Work out the finished part from the listing and answer in its coordinate system (mm). A direction names the side the tool comes from. Round coordinates to 2 decimals unless told otherwise and drop trailing zeros. Loops run counter-clockwise (first coordinate to the right, second up) from the corner with the lowest first, then second, coordinate; pieces in that order, holes last.
from build123d import *

# Parameters (mm, degrees)
F0_W     = 19.05
F0_H     = 76.2
F1_DEPTH = 19.05


with BuildPart() as f1:
    # F0 (on Right) → F1 (new body)
    with BuildSketch(Plane.YZ):
        Polygon((0, 34.459569), (0, 0), (457.2, 0), (457.2, 34.459569), (457.2, 110.659569), (457.2, 212.259569), (457.2, 288.459569), (457.2, 390.059569), (457.2, 466.259569), (457.2, 609.6), (0, 609.6), (0, 466.259569), (0, 390.059569), (0, 288.459569), (0, 212.259569), (0, 110.659569), align=None)
        with Locations((-9.525, 72.559569)):
            Rectangle(F0_W, F0_H)
        with Locations((466.725, 72.559569)):
            Rectangle(F0_W, F0_H)
        with Locations((-9.525, 250.359569)):
            Rectangle(F0_W, F0_H)
        with Locations((466.725, 250.359569)):
            Rectangle(F0_W, F0_H)
        with Locations((-9.525, 428.159569)):
            Rectangle(F0_W, F0_H)
        with Locations((466.725, 428.159569)):
            Rectangle(F0_W, F0_H)
    extrude(amount=F1_DEPTH)


solid = f1.part
Item 1: Determine the mould class of faces 6 (the face through (9, 457.2, 537)), 7 (the face through (9, 467, 212.26)), 8 (the face through (9, 232, 609.6)), 9 (the face through (9, 225, 0)) for opening direction Z: pulls with the +Z half, pulls with the -Z half, needs draft (parallel to the pull), parting line crosses it, or undercut.
Item 2: A straight line is drawn through the part: line 1 (Y direction, x = 17.25, z = 346). Find the intervals that lie inside material, in ascending order.
Item 3: For faces 1 (the face through (9, 457.2, 161)), 2 (the face through (9, -19.05, 250)), 3 (the face through (9, -10, 390.06)), 4 (the face through (9, 0, 17)), 5 (the face through (9, 467, 34.46)), determine the directions among +Z, -Z, +X, -X, +Y, -Y from which every point of the face is accessible in a straight line to the end or side of a thin tool.
Item 4: Section A-A, the plane x = 8 is taken. Give the vertices of the cut face in (y, z).
Item 5: Each of these flat-tipped pins is pushed along its axis until it touches: P1, Ø5.5, axis at x = 11.5, y = -11, coming from the +Z side; P2, Ø9.5, axis at x = 14, y = 471, coming from the -Z side; P3, Ø2, axis at y = 368, z = 153, coming from the -X side; P4, Ø5.5, axis at x = 7.5, z = 167.5, coming from the +Y side. Where does it stop, or does it pass through?
Item 6: Section B-B, the plane z = 501 is taken. Give the vertices of the cut face in (x, y), plus the area to 3 significant figures.
Answer below:
1. face 6: needs draft
1. face 7: undercut
1. face 8: pulls with the +Z half
1. face 9: pulls with the -Z half
2. line 1: y = 0 to 457.2
3. face 1: +X, -X, +Y
3. face 2: +Z, -Z, +X, -X, -Y
3. face 3: +X, -X, -Y
3. face 4: -Z, +X, -X, -Y
3. face 5: -Z, +X, -X, +Y
4. outline: (-19.05, 34.46) - (0, 34.46) - (0, 0) - (457.2, 0) - (457.2, 34.46) - (476.25, 34.46) - (476.25, 110.66) - (457.2, 110.66) - (457.2, 212.26) - (476.25, 212.26) - (476.25, 288.46) - (457.2, 288.46) - (457.2, 390.06) - (476.25, 390.06) - (476.25, 466.26) - (457.2, 466.26) - (457.2, 609.6) - (0, 609.6) - (0, 466.26) - (-19.05, 466.26) - (-19.05, 390.06) - (0, 390.06) - (0, 288.46) - (-19.05, 288.46) - (-19.05, 212.26) - (0, 212.26) - (0, 110.66) - (-19.05, 110.66) - close
5. P1: stops at z = 466.26
5. P2: stops at z = 34.46
5. P3: stops at x = 0
5. P4: stops at y = 457.2
6. outline: (0, 0) - (19.05, 0) - (19.05, 457.2) - (0, 457.2) - close
6. area: 8,710 mm2
